```python
from build123d import *

# Parameters (mm, degrees)
F0_W     = 25
F0_H     = 50
F1_DEPTH = 25


with BuildPart() as f1:
    # F0 (on Right) → F1 (new body)
    with BuildSketch(Plane.YZ):
        Polygon((-200, 0), (0, 0), (0, 25), (-25, 25), (-200, 25), align=None)
        with Locations((-12.5, 50)):
            Rectangle(F0_W, F0_H)
        Polygon((-25, 75), (-200, 25), (-25, 25), align=None)
    extrude(amount=F1_DEPTH)


solid = f1.part
```
Work out the finished part from the listing and answer in its coordinate system (mm). Coordinates: 2 decimals unless noted, no trailing zeros. Write each loop counter-clockwise with the first axis right and the second up, starting at its lowest first coordinate (ties: lowest second). Pieces come first, ordered by that corner, then holes. Notation, with made-up numbers: (66, 84.5) - (113, 84.5) arc R21 ccw to (113, 110.5) - close; hole circle Ø4 at (74.25, 60.5). An arc over 180 degrees is marked (long way). Answer as a JSON object with one key per item and string values.
Q1. Find section A-A (x = 12.25). Write down the section's boundary in (y, z), plus the area to 3 significant figures.
Results list:
{"outline": "(-200, 0) - (0, 0) - (0, 75) - (-25, 75) - (-200, 25) - close", "area": "10,600 mm^2"}
Q2. Consider L1, parallel to Z at x = 23.5, y = -191; L2, parallel to Z at x = 14.5, y = -120. Determine where each line is inside the solid, lowest interval first. Write a range as from..to.
Results list:
{"L1": "z = 0..27.57", "L2": "z = 0..47.86"}
Q3. Find section C-C (z = 52.5). Write down the section's boundary in (x, y), plus the area to 3 significant figures.
Results list:
{"outline": "(0, -103.75) - (25, -103.75) - (25, 0) - (0, 0) - close", "area": "2,590 mm^2"}
Q4. Find section B-B (y = -56.5). Write down the section's boundary in (x, z).
Results list:
{"outline": "(0, 0) - (25, 0) - (25, 66) - (0, 66) - close"}
Q5. Given pin 1 Ø10 at (x, y) = (5.5, -115.5) entering from +Z, flat-ended and moving along its own axis, determine where the tip first touches the part or whether it passes through.
Results list:
{"pin 1": "stops at z = 50.57"}
